CAD build for the part. Positions are in the model's coordinates, mm. A direction names the side the tool comes from. Round coordinates to 2 decimals unless told otherwise and drop trailing zeros. Loops run counter-clockwise (first coordinate to the right, second up) from the corner with the lowest first, then second, coordinate; pieces in that order, holes last. Notation, with made-up numbers: M -15.75,10.25 L 23.25,10.25 A35 cw 23.25,43.25 Z; hole C 57,12.5 d9. An arc over 180 degrees is marked long. Use one line per item in the form item = value.
from build123d import *

# Parameters (mm, degrees)
F0_R     = 22.5
F1_DEPTH = 4
F2_R     = 17
F3_DEPTH = 4
F5_DEPTH = 1.75
F6_R     = 1.6
F7_DEPTH = 4


with BuildPart() as f1:
    # F0 (on Top) → F1 (new body)
    with BuildSketch(Plane.XY):
        Circle(F0_R)
    extrude(amount=F1_DEPTH)

    # F2 (on face) → F3 (cut)
    with BuildSketch(Plane.XY.offset(4)):
        Circle(F2_R)
    extrude(amount=-F3_DEPTH, mode=Mode.SUBTRACT)

    # F4 (on face) → F5 (cut)
    with BuildSketch(Plane.XY.offset(4)):
        with BuildLine():
            Line((-6.6176470588, 21.5048075417), (-5, 16.2480768093))
            ThreePointArc((-5, 16.2480768093), (0, 17), (5, 16.2480768093))
            Line((5, 16.2480768093), (6.6176470588, 21.5048075417))
            ThreePointArc((6.6176470588, 21.5048075417), (0, 22.5), (-6.6176470588, 21.5048075417))
        make_face()
        with BuildLine():
            Line((-16.5712472795, -3.7939113857), (-21.932533164, -5.0213533046))
            ThreePointArc((-21.932533164, -5.0213533046), (-19.4855715851, -11.25), (-15.3148861052, -16.4834542371))
            Line((-15.3148861052, -16.4834542371), (-11.5712472795, -12.4541654236))
            ThreePointArc((-11.5712472795, -12.4541654236), (-14.7224318643, -8.5), (-16.5712472795, -3.7939113857))
        make_face()
        with BuildLine():
            Line((11.5712472795, -12.4541654236), (15.3148861052, -16.4834542371))
            ThreePointArc((15.3148861052, -16.4834542371), (19.4855715851, -11.25), (21.932533164, -5.0213533046))
            Line((21.932533164, -5.0213533046), (16.5712472795, -3.7939113857))
            ThreePointArc((16.5712472795, -3.7939113857), (14.7224318643, -8.5), (11.5712472795, -12.4541654236))
        make_face()
    extrude(amount=-F5_DEPTH, mode=Mode.SUBTRACT)

    # F6 (on face) → F7 (cut)
    with BuildSketch(Plane.XY.offset(4)):
        with Locations((0, -20)):
            Circle(F6_R)
        with Locations((17.3205080757, 10)):
            Circle(F6_R)
        with Locations((-17.3205080757, 10)):
            Circle(F6_R)
    extrude(amount=-F7_DEPTH, mode=Mode.SUBTRACT)


solid = f1.part
1. Cut at D-D on y = 10. Write the cut outline in (x, z), and give its area (3 significant figures).
Completed:
outline = M -20.16,0 L -18.92,0 L -18.92,4 L -20.16,4 Z; M -15.72,0 L -13.75,0 L -13.75,4 L -15.72,4 Z; M 13.75,0 L 15.72,0 L 15.72,4 L 13.75,4 Z; M 18.92,0 L 20.16,0 L 20.16,4 L 18.92,4 Z
area = 25.7 mm2
2. Cut at A-A on z = 2.95. Write the cut outline in (x, y), and give its area (3 significant figures).
Completed:
outline = M -21.93,-5.02 L -16.57,-3.79 A17 cw -5,16.25 L -6.62,21.5 A22.5 ccw Z; M -15.31,-16.48 A22.5 ccw 15.31,-16.48 L 11.57,-12.45 A17 cw -11.57,-12.45 Z; M 5,16.25 A17 cw 16.57,-3.79 L 21.93,-5.02 A22.5 ccw 6.62,21.5 Z; hole C -17.32,10 d3.2; hole C 0,-20 d3.2; hole C 17.32,10 d3.2
area = 464 mm2
3. Cut at B-B on y = 0. Write the cut outline in (x, z).
Completed:
outline = M -22.5,0 L -17,0 L -17,4 L -22.5,4 Z; M 17,0 L 22.5,0 L 22.5,4 L 17,4 Z
4. Tool access for faces 4 (the face through (-13.47, -14.5, 3.14)), 5 (the face through (5.797, 18.84, 3.137)), 6 (the face through (-19.21, -4.4, 3.14)), 7 (the face through (13.417, -14.441, 3.137)), 8 (the face through (5, -17, 0)): list every direction of +Z, -Z, +X, -X, +Y, -Y with a clear straight run to the whole face (end or side of a thin tool).
Completed:
face_4 = +Z, -X
face_5 = +Z, +Y
face_6 = +Z, -Y
face_7 = +Z, +X
face_8 = -Z, +X, -X, +Y, -Y
5. Drop flat-ended pins along their axis: P1, Ø11.5, axis at x = -17.5, y = -7.5, coming from the +Z side; P2, Ø3, axis at x = -3.5, y = 18.5, coming from the +Z side; P3, Ø1, axis at y = 7, z = 3, coming from the -X side. Give the stop position or say it passes through.
Completed:
P1 = 4
P2 = 2.25
P3 = -21.54
6. Cut at C-C on x = 0. Write the cut outline in (y, z).
Completed:
outline = M -22.5,0 L -21.6,0 L -21.6,4 L -22.5,4 Z; M -18.4,0 L -17,0 L -17,4 L -18.4,4 Z; M 17,0 L 22.5,0 L 22.5,2.25 L 17,2.25 Z
7. Pull direction Y, two halves, no side cores. Call faces 1 (the face through (-2.213, 16.855, 2.028)), 2 (the face through (-5.82, 18.91, 3.14)), 3 (the face through (-0.2, -17.4, 4)): +Y half, -Y half, draft (parallel to the pull), parting line (faces both ways), or undercut.
Completed:
face_1 = undercut
face_2 = +Y half
face_3 = draft
8. Probe line 1 along Y through (x, z) = (0, 0.85); line 2 along Y through (x, z) = (0, 3.05); line 3 along Y through (x, z) = (1, 1.6). List the from-to ranges inside material, lowest first. Write a range as from..to.
Completed:
line_1 = -22.5..-21.6, -18.4..-17, 17..22.5
line_2 = -22.5..-21.6, -18.4..-17
line_3 = -22.48..-21.25, -18.75..-16.97, 16.97..22.48
